```python
from build123d import *

# Parameters (mm, degrees)
BOSS_EXTRUDE1_DEPTH = 16
SKETCH2_R           = 2.5
BOSS_EXTRUDE2_DEPTH = 1.3
SKETCH3_W           = 10
SKETCH3_H           = 12
BOSS_EXTRUDE3_DEPTH = 9
SKETCH4_R           = 2
BOSS_EXTRUDE4_DEPTH = 0.7
SKETCH5_R           = 1.5
BOSS_EXTRUDE5_DEPTH = 9
SKETCH6_W           = 5.348549536
SKETCH6_H           = 1.415696151
CUT_EXTRUDE1_DEPTH  = 8.9


with BuildPart() as part:
    # Sketch1 → Boss-Extrude1 (new body)
    with BuildSketch(Plane.XY):
        with BuildLine():
            Line((-5, -1), (-5, 1))
            ThreePointArc((-5, 1), (0, 6), (5, 1))
            Line((5, 1), (5, -1))
            ThreePointArc((5, -1), (0, -6), (-5, -1))
        make_face()
    extrude(amount=BOSS_EXTRUDE1_DEPTH)

    # Sketch2 → Boss-Extrude2 (add)
    with BuildSketch(Plane(origin=(0, 0, 0), x_dir=(-1, 0, 0), z_dir=(0, 0, -1))):
        Circle(SKETCH2_R)
    extrude(amount=BOSS_EXTRUDE2_DEPTH)

    # Sketch3 → Boss-Extrude3 (add)
    with BuildSketch(Plane.XY.offset(16)):
        Rectangle(SKETCH3_W, SKETCH3_H)
    extrude(amount=BOSS_EXTRUDE3_DEPTH)

    # Sketch4 → Boss-Extrude4 (add)
    with BuildSketch(Plane.XY.offset(25)):
        Circle(SKETCH4_R)
    extrude(amount=BOSS_EXTRUDE4_DEPTH)

    # Sketch5 → Boss-Extrude5 (add)
    with BuildSketch(Plane.XY.offset(25.7)):
        Circle(SKETCH5_R)
    extrude(amount=BOSS_EXTRUDE5_DEPTH)

    # Sketch6 → Cut-Extrude1 (cut)
    with BuildSketch(Plane.XY.offset(34.7)):
        with Locations((0, -1.707848076)):
            Rectangle(SKETCH6_W, SKETCH6_H)
    extrude(amount=-CUT_EXTRUDE1_DEPTH, mode=Mode.SUBTRACT)


solid = part.part
```
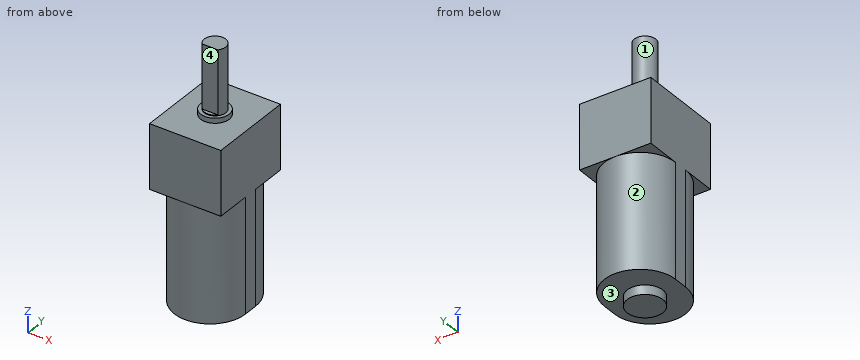
CAD build for the part. Positions are in the model's coordinates, mm. Face numbers are marked on the shaded views. A direction names the side the tool comes from. Round coordinates to 2 decimals unless told otherwise and drop trailing zeros. Order: outer loops, then holes, each group sorted by start corner. A loop starts at its lowest first (then second) coordinate and runs counter-clockwise, first axis right, second up. Notation, with made-up numbers: (39, 25.25) - (75, 25.25) arc R35 ccw to (75, 57.25) - close; hole circle Ø8 at (-38, -39.5). An arc over 180 degrees is marked (long way). Answer as CSV lines item,"result". Start each with the question number.
1. Saw through at D-D, the plane x = -3.75. Write the cut outline in (y, z), and give its area (3 significant figures).
2. Pin check, flat tips, straight feed: pin 1 (6 mm diameter, centred on y = -3.5, z = 29, fed in from +X); pin 2 (1.5 mm diameter, centred on x = -2, y = 3, fed in from -Z); pin 3 (1.1 mm diameter, centred on x = 0, z = 31, fed in from -Y). Stop position of each tip, or through.
3. Saw through at A-A, the plane x = 4. Write the cut outline in (y, z).
4. Saw through at C-C, the plane z = 11.5. Write the cut outline in (x, y).
5. Saw through at B-B, the plane y = 0. Write the cut outline in (x, z), and give its area (3 significant figures).
6. Tool access for the marked faces 1, 2, 3 and 4: list every direction of +Z, -Z, +X, -X, +Y, -Y with a clear straight run to the whole face (end or side of a thin tool).
7. Drill centre lines: L1, parallel to Z at x = 4, y = -3.5; L2, parallel to Y at x = -3, z = 11.5; L3, parallel to Z at x = 0.75, y = 2. Where is each one in solid material? Low to high. Write a range as [from, to].
Model answer:
1,outline,"(-6, 16) - (-4.31, 16) - (-4.31, 0) - (4.31, 0) - (4.31, 16) - (6, 16) - (6, 25) - (-6, 25) - close"
1,area,"246 mm²"
2,pin 1,"stops at x = 1.41"
2,pin 2,"stops at z = 0"
2,pin 3,"stops at y = -1"
3,outline,"(-6, 16) - (-4, 16) - (-4, 0) - (4, 0) - (4, 16) - (6, 16) - (6, 25) - (-6, 25) - close"
4,outline,"(-5, -1) arc R5 ccw to (5, -1) - (5, 1) arc R5 ccw to (-5, 1) - close"
5,outline,"(-5, 0) - (-2.5, 0) - (-2.5, -1.3) - (2.5, -1.3) - (2.5, 0) - (5, 0) - (5, 25) - (2, 25) - (2, 25.7) - (1.5, 25.7) - (1.5, 34.7) - (-1.5, 34.7) - (-1.5, 25.7) - (-2, 25.7) - (-2, 25) - (-5, 25) - close"
5,area,"286 mm²"
6,face 1,"+Z"
6,face 2,"-Z, +Y"
6,face 3,"-Z"
6,face 4,"+Z, +X, -X, -Y"
7,L1,"z = [0, 25]"
7,L2,"y = [-5, 5]"
7,L3,"z = [-1.3, 25]"
